from build123d import *

# Parameters (mm, degrees)
F1_DEPTH = 70
F3_START = -25
F2_R     = 150
F3_DEPTH = 50


with BuildPart() as f1:
    # F0 (on Front) → F1 (new body)
    with BuildSketch(Plane.XZ):
        with BuildLine():
            ThreePointArc((-21, -0.4), (-20, 0.1), (-19, -0.4))
            ThreePointArc((-19, -0.4), (-18, -0.9), (-17, -0.4))
            ThreePointArc((-17, -0.4), (-16, 0.1), (-15, -0.4))
            ThreePointArc((-15, -0.4), (-14, -0.9), (-13, -0.4))
            ThreePointArc((-13, -0.4), (-12, 0.1), (-11, -0.4))
            ThreePointArc((-11, -0.4), (-10, -0.9), (-9, -0.4))
            ThreePointArc((-9, -0.4), (-8, 0.1), (-7, -0.4))
            ThreePointArc((-7, -0.4), (-6, -0.9), (-5, -0.4))
            ThreePointArc((-5, -0.4), (-4, 0.1), (-3, -0.4))
            ThreePointArc((-3, -0.4), (-2, -0.9), (-1, -0.4))
            ThreePointArc((-1, -0.4), (0, 0.1), (1, -0.4))
            ThreePointArc((1, -0.4), (2, -0.9), (3, -0.4))
            ThreePointArc((3, -0.4), (4, 0.1), (5, -0.4))
            ThreePointArc((5, -0.4), (6, -0.9), (7, -0.4))
            ThreePointArc((7, -0.4), (8, 0.1), (9, -0.4))
            ThreePointArc((9, -0.4), (10, -0.9), (11, -0.4))
            ThreePointArc((11, -0.4), (12, 0.1), (13, -0.4))
            ThreePointArc((13, -0.4), (14, -0.9), (15, -0.4))
            ThreePointArc((15, -0.4), (16, 0.1), (17, -0.4))
            ThreePointArc((17, -0.4), (18, -0.9), (19, -0.4))
            ThreePointArc((19, -0.4), (20, 0.1), (21, -0.4))
            ThreePointArc((21, -0.4), (22, -0.9), (23, -0.4))
            ThreePointArc((23, -0.4), (24, 0.1), (25, -0.4))
            Line((25, -0.4), (25, 0.4))
            ThreePointArc((25, 0.4), (24, 0.9), (23, 0.4))
            ThreePointArc((23, 0.4), (22, -0.1), (21, 0.4))
            ThreePointArc((21, 0.4), (20, 0.9), (19, 0.4))
            ThreePointArc((19, 0.4), (18, -0.1), (17, 0.4))
            ThreePointArc((17, 0.4), (16, 0.9), (15, 0.4))
            ThreePointArc((15, 0.4), (14, -0.1), (13, 0.4))
            ThreePointArc((13, 0.4), (12, 0.9), (11, 0.4))
            ThreePointArc((11, 0.4), (10, -0.1), (9, 0.4))
            ThreePointArc((9, 0.4), (8, 0.9), (7, 0.4))
            ThreePointArc((7, 0.4), (6, -0.1), (5, 0.4))
            ThreePointArc((5, 0.4), (4, 0.9), (3, 0.4))
            ThreePointArc((3, 0.4), (2, -0.1), (1, 0.4))
            ThreePointArc((1, 0.4), (0, 0.9), (-1, 0.4))
            ThreePointArc((-1, 0.4), (-2, -0.1), (-3, 0.4))
            ThreePointArc((-3, 0.4), (-4, 0.9), (-5, 0.4))
            ThreePointArc((-5, 0.4), (-6, -0.1), (-7, 0.4))
            ThreePointArc((-7, 0.4), (-8, 0.9), (-9, 0.4))
            ThreePointArc((-9, 0.4), (-10, -0.1), (-11, 0.4))
            ThreePointArc((-11, 0.4), (-12, 0.9), (-13, 0.4))
            ThreePointArc((-13, 0.4), (-14, -0.1), (-15, 0.4))
            ThreePointArc((-15, 0.4), (-16, 0.9), (-17, 0.4))
            ThreePointArc((-17, 0.4), (-18, -0.1), (-19, 0.4))
            ThreePointArc((-19, 0.4), (-20, 0.9), (-21, 0.4))
            ThreePointArc((-21, 0.4), (-22, -0.1), (-23, 0.4))
            ThreePointArc((-23, 0.4), (-24, 0.9), (-25, 0.4))
            Line((-25, 0.4), (-25, -0.4))
            ThreePointArc((-25, -0.4), (-24, 0.1), (-23, -0.4))
            ThreePointArc((-23, -0.4), (-22, -0.9), (-21, -0.4))
        make_face()
    extrude(amount=F1_DEPTH)

    # F2 (on Top) → F3 (intersect)
    with BuildSketch(Plane.XY.offset(F3_START)):
        with Locations((48, -150)):
            Circle(F2_R)
    extrude(amount=F3_DEPTH, mode=Mode.INTERSECT)


solid = f1.part
Design review of the part built by this model. Coordinates are the model's own, in mm. Coordinates: 2 decimals unless noted, no trailing zeros. Loops run counter-clockwise (first coordinate to the right, second up) from the corner with the lowest first, then second, coordinate; pieces in that order, holes last.
Item 1: Add section B-B (x = -10). Write out the cut boundary in (y, z), and give its area (3 significant figures).
Completed:
outline: (-70, -0.9) - (-11.67, -0.9) - (-11.67, -0.1) - (-70, -0.1) - close
area: 46.7 mm2
Item 2: Wall thickness on L1, parallel to Y at x = 15, z = -0.1; L2, parallel to Z at x = 19, y = -41; L3, parallel to Z at x = 4, y = -46.5: over which ranges is each line inside the solid? List them lowest first.
Completed:
L1: y = -70 to -3.68
L2: z = -0.4 to 0.4
L3: z = 0.1 to 0.9
Item 3: Clearance check with a flat-ended pin moving along its axis: pin 1 (1.5 mm diameter, centred on x = -13.5, y = -57.5, fed in from -Z). State where the tip first meets the part, or that it passes through.
Completed:
pin 1: stops at z = -0.9
Item 4: Add section A-A (x = 14). Write out the cut boundary in (y, z), and give its area (3 significant figures).
Completed:
outline: (-70, -0.9) - (-3.9, -0.9) - (-3.9, -0.1) - (-70, -0.1) - close
area: 52.9 mm2
